Could you check a few things on this model? Use its own coordinates, in mm. A direction names the side the tool comes from. Give positions to 0.01 mm unless a question says otherwise; leave off trailing zeros. Loops run counter-clockwise (first coordinate to the right, second up) from the corner with the lowest first, then second, coordinate; pieces in that order, holes last.
1. I need wall thicknesses on line 1 along Z through (x, y) = (-7.05, -27.5); line 2 along X through (y, z) = (2.5, -3.75) (3 decimals); line 3 along Y through (x, z) = (-14.55, 0). Which ranges of each line are inside material? Lowest first, please.
2. Thinking about a two-plate mould opening in Z: for faces 1 (the cylindrical face through (-14.265, -2.685, 0.596)), 2 (the flat face through (-9, -15, -7.5)), 3 (the flat face through (-15.875, 3, -2)), which applies, +Z half, -Z half, draft (parallel to the pull), parting line (faces both ways), or undercut?
3. Imagine slicing it at B-B (y = 0). List the corners of the cut face in (x, z) for me (3 decimals), plus the area to 3 significant figures.
4. Imagine slicing it at C-C (z = 0). Count the separate pieces of the cut face and the enclosed holes in it, plus the area to 3 significant figures.
5. For faces 4 (the cylindrical face through (-14.31, 6.64, -6.6)), 5 (the flat face through (-8.587, -28, -3)), 6 (the flat face through (-12.7, 3, 0)), which set-ups out of +Z, -Z, +X, -X, +Y, -Y let a thin tool reach every point of the face, with its end or its side?
6. Imagine slicing it at A-A (y = -27.5). List the corners of the cut face in (x, z) for me, plus the area to 4 significant figures.
7. For P1, Ø4, axis at x = -10, z = 4.5, coming from the +Y side; P2, Ø1.5, axis at y = -11, z = -3.5, coming from the +X side; P3, Ø8.5, axis at y = 1.5, z = 2, coming from the +X side, each with a flat end and sliding along its axis, tell me the tip position at first contact or that it passes through.
```python
from build123d import *

# Parameters (mm, degrees)
FILLET1_R               = 7
M5_CLEARANCE_HOLE1_D    = 5.5
CUT_EXTRUDE1_DEPTH      = 37.52886072966826
CUT_EXTRUDE1_DEPTH_BACK = 37.52886072966826
SKETCH3_R               = 2.4999999999999996
FILLET2_R               = 3


with BuildPart() as part:
    # Sweep1: sweep along a path in Sketch1
    with BuildLine(Plane.XY) as sweep1_path:
        Line((-14.2875, 7.5), (-14.2875, -7.5))
        ThreePointArc((-14.2875, -7.5), (-8.903716825795872, -12.735560659438995), (-7.000000000000001, -20))
        Line((-7.000000000000001, -20), (-6.999999999999999, -35))
    # Sketch2 → Sweep1 (sweep)
    with BuildSketch(Plane(origin=(0, 0, 0), x_dir=(1, 0, 0), z_dir=(0, 1, 0))):
        Polygon((-12.699999999999996, -7.499999999999996), (-15.874999999999996, -7.499999999999996), (-15.874999999999996, 7.500000000000004), (-12.699999999999996, 7.500000000000005), align=None)
    sweep(path=sweep1_path.line, transition=Transition.RIGHT)

    # Fillet1
    fillet1_edges = [part.edges().sort_by_distance(p)[0] for p in [
        (-15.874999999999996, -8.441785890670294, -1.599e-14),
        (-12.699999999999996, -6.5917812273426035, -7.11e-15),
    ]]
    fillet(fillet1_edges, radius=FILLET1_R)

    # M5 Clearance Hole1 (through all)
    with Locations(Plane.ZY.offset(15.874999999999996)):
        with Locations((0, 0)):
            Hole(M5_CLEARANCE_HOLE1_D / 2)

    # Sketch3 → Cut-Extrude1 (cut, two sides: drawn at the far end of the back side and taken through both)
    with BuildSketch(Plane.ZY.offset(8.587500000000007).offset(-CUT_EXTRUDE1_DEPTH_BACK)):
        with Locations(Location((0, -27.500000000000004, 0), (0, 0, 270))):
            Circle(SKETCH3_R)
    extrude(amount=CUT_EXTRUDE1_DEPTH + CUT_EXTRUDE1_DEPTH_BACK, mode=Mode.SUBTRACT)

    # Fillet2
    fillet2_edges = [part.edges().sort_by_distance(p)[0] for p in [
        (-14.287499999999996, 7.5, 7.499999999999996),
        (-14.287499999999996, 7.5, -7.500000000000005),
    ]]
    fillet(fillet2_edges, radius=FILLET2_R)


solid = part.part
```
Derived:
1. line 1: z = -7.5 to -2.5, 2.5 to 7.5
1. line 2: x = -15.875 to -12.7
1. line 3: y = -8.72 to -2.75, 2.75 to 7.5
2. face 1: undercut
2. face 2: -Z half
2. face 3: draft
3. outline: (-15.875, -7.5) - (-12.7, -7.5) - (-12.7, -2.75) - (-15.875, -2.75) - close; (-15.875, 2.75) - (-12.7, 2.75) - (-12.7, 7.5) - (-15.875, 7.5) - close
3. area: 30.2 mm2
4. separate pieces: 3
4. enclosed holes: 0
4. area: 110 mm2
5. face 4: -Z, +X, -X, +Y
5. face 5: +Z, -Z, -X, -Y
5. face 6: +Z, -Z, +X, +Y
6. outline: (-8.59, -7.5) - (-5.41, -7.5) - (-5.41, -2.5) - (-8.59, -2.5) - close; (-8.59, 2.5) - (-5.41, 2.5) - (-5.41, 7.5) - (-8.59, 7.5) - close
6. area: 31.75 mm2
7. P1: stops at y = -6.22
7. P2: stops at x = -7.64
7. P3: stops at x = -12.7
